```python
from build123d import *

# Parameters (mm, degrees)
F0_R     = 4
F1_DEPTH = 38
F0_R_2   = 6
F2_DEPTH = 6
F3_SIZE  = 1.2
F4_R     = 1.5
F5_DEPTH = 4


with BuildPart() as f1:
    # F0 (on Right) → F1 (new body)
    with BuildSketch(Plane.YZ):
        Circle(F0_R)
    extrude(amount=F1_DEPTH)

    # F0 (on Right) → F2 (join)
    with BuildSketch(Plane.YZ):
        Circle(F0_R_2)
        Circle(F0_R, mode=Mode.SUBTRACT)
    extrude(amount=F2_DEPTH)

    # F3
    f3_edges = [f1.edges().sort_by_distance(p)[0] for p in [
        (0, -6, 0),
    ]]
    chamfer(f3_edges, length=F3_SIZE)

    # F4 (on Front) → F5 (cut, symmetric)
    with BuildSketch(Plane.XZ):
        with Locations((35.5, 0)):
            Circle(F4_R)
    extrude(amount=F5_DEPTH, both=True, mode=Mode.SUBTRACT)


solid = f1.part
```
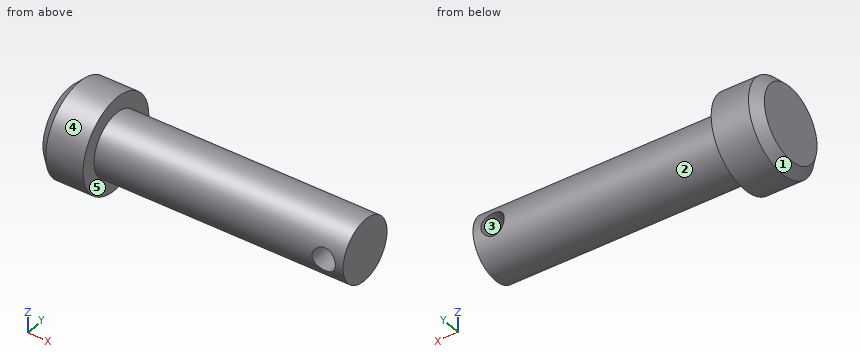
Input: part model. Units: mm. Frame: model coordinates. Face numbers are marked on the shaded views. A direction names the side the tool comes from. Give positions to 0.01 mm unless a question says otherwise; leave off trailing zeros. Write each loop counter-clockwise with the first axis right and the second up, starting at its lowest first coordinate (ties: lowest second). Pieces come first, ordered by that corner, then holes. Notation, with made-up numbers: (32, 28) - (55, 28) arc R12 cw to (55, 36) - close; hole circle Ø6 at (-26.75, 82.5). An arc over 180 degrees is marked (long way). Write item = value, one per line. Start each with the question number.
1) Cut plane B-B (z = 0). Return loops of the section in (x, y), and give its area (3 significant figures).
2) Material intervals for L1, parallel to X at y = -1, z = 0; L2, parallel to Z at x = 12, y = 0; L3, parallel to Z at x = 35.5, y = 1, sorted ascending. Write a range as [from, to].
3) Draft query along Z for the marked faces 3, 4 and 5. Return one class per face: pulls with the +Z half, pulls with the -Z half, needs draft (parallel to the pull), parting line crosses it, or undercut.
4) Cut plane A-A (y = 0). Return loops of the section in (x, z).
5) Pin query (flat end, axial travel): pin 1 (1 mm diameter, centred on x = 19, z = 1.5, fed in from +Y); pin 2 (4 mm diameter, centred on x = 31.5, z = 1.5, fed in from -Y); pin 3 (3 mm diameter, centred on x = 13.5, y = -2, fed in from +Z). Return the tip coordinate at first contact, or that it passes through.
6) Reachability of the marked faces 1 and 2 from +Z, -Z, +X, -X, +Y, -Y: full face, straight path, thin tool, end or side. Return the list, or none.
7) Cut plane C-C (x = 35.5). Return loops of the section in (y, z).
8) Cut plane D-D (x = 4). Return loops of the section in (y, z).
Answers follow:
q1.outline = (0, -4.8) - (1.2, -6) - (6, -6) - (6, -4) - (34, -4) - (34, 4) - (6, 4) - (6, 6) - (1.2, 6) - (0, 4.8) - close; (37, -4) - (38, -4) - (38, 4) - (37, 4) - close
q1.area = 303 mm^2
q2.L1 = [0, 34], [37, 38]
q2.L2 = [-4, 4]
q2.L3 = [-3.87, -1.5], [1.5, 3.87]
q3.face_3 = undercut
q3.face_4 = parting line crosses it
q3.face_5 = needs draft
q4.outline = (0, -4.8) - (1.2, -6) - (6, -6) - (6, -4) - (38, -4) - (38, 4) - (6, 4) - (6, 6) - (1.2, 6) - (0, 4.8) - close; hole circle Ø3 at (35.5, 0)
q5.pin_1 = 3.87
q5.pin_2 = -4
q5.pin_3 = 3.97
q6.face_1 = -X
q6.face_2 = +X
q7.outline = (-3.71, -1.5) arc R4 ccw to (3.71, -1.5) - close; (-3.71, 1.5) - (3.71, 1.5) arc R4 ccw to start
q8.outline = circle Ø12 at (0, 0)
